Read the model definition and answer for the solid it produces. Units are mm, in the model's axes. Face numbers are marked on the shaded views. A direction names the side the tool comes from. Coordinates: 2 decimals unless noted, no trailing zeros. Loops run counter-clockwise (first coordinate to the right, second up) from the corner with the lowest first, then second, coordinate; pieces in that order, holes last.
from build123d import *

# Parameters (mm, degrees)
SKETCH_1_R          = 4.5
SKETCH_1_R_2        = 3
EXTRUDE_1_DEPTH     = 2
SKETCH_2_R          = 10
SKETCH_2_R_2        = 1.65
EXTRUDE_2_DEPTH     = 2.5
SKETCH_3_R          = 1.5
CUT_EXTRUDE_1_DEPTH = 2.5


with BuildPart() as part:
    # 草图1 → 凸台-拉伸1 (new body)
    with BuildSketch(Plane.XY):
        Circle(SKETCH_1_R)
        Circle(SKETCH_1_R_2, mode=Mode.SUBTRACT)
    extrude(amount=EXTRUDE_1_DEPTH)

    # 草图2 → 凸台-拉伸2 (add)
    with BuildSketch(Plane(origin=(0, 0, 0), x_dir=(-1, 0, 0), z_dir=(0, 0, -1))):
        Circle(SKETCH_2_R)
        Circle(SKETCH_2_R_2, mode=Mode.SUBTRACT)
    extrude(amount=EXTRUDE_2_DEPTH)

    # 草图3 → 切除-拉伸1 (cut)
    with BuildSketch(Plane(origin=(0, 0, -2.5), x_dir=(-1, 0, 0), z_dir=(0, 0, -1))):
        with Locations((7, 0)):
            Circle(SKETCH_3_R)
        with Locations((0, -7)):
            Circle(SKETCH_3_R)
        with Locations((-7, 0)):
            Circle(SKETCH_3_R)
        with Locations((0, 7)):
            Circle(SKETCH_3_R)
    extrude(amount=-CUT_EXTRUDE_1_DEPTH, mode=Mode.SUBTRACT)


solid = part.part
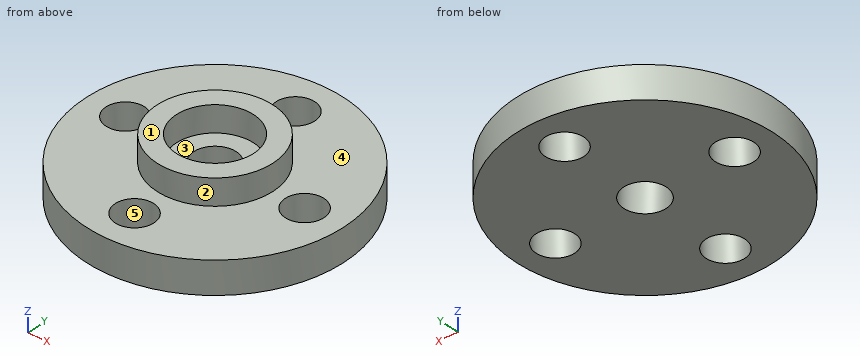
Item 1: A cutting plane is placed at B-B on y = 1.25. Determine the outline of the cut face in (x, z).
Numbers:
outline: (-9.92, -2.5) - (-7.83, -2.5) - (-7.83, 0) - (-9.92, 0) - close; (-6.17, -2.5) - (-1.08, -2.5) - (-1.08, 0) - (-2.73, 0) - (-2.73, 2) - (-4.32, 2) - (-4.32, 0) - (-6.17, 0) - close; (1.08, -2.5) - (6.17, -2.5) - (6.17, 0) - (4.32, 0) - (4.32, 2) - (2.73, 2) - (2.73, 0) - (1.08, 0) - close; (7.83, -2.5) - (9.92, -2.5) - (9.92, 0) - (7.83, 0) - close
Item 2: A cutting plane is placed at D-D on z = 0.4. Determine the outline of the cut face in (x, y).
Numbers:
outline: circle Ø9 at (0, 0); hole circle Ø6 at (0, 0)
Item 3: Given pin 1 (2 mm diameter, centred on x = 4, z = 0, fed in from +Y); pin 2 (4 mm diameter, centred on x = 6.5, y = 6.5, fed in from +Z); pin 3 (1.8 mm diameter, centred on x = -7, y = 0, fed in from -Z), each flat-ended and moving along its own axis, determine where each tip first touches the part or whether it passes through.
Numbers:
pin 1: stops at y = 9.54
pin 2: stops at z = 0
pin 3: passes through
Item 4: Determine the mould class of the marked faces 1, 2 and 3 for opening direction Y: released by +Y, released by -Y, zero draft, split by the parting line, or undercut.
Numbers:
face 1: zero draft
face 2: split by the parting line
face 3: undercut
Item 5: A cutting plane is placed at C-C on y = 7.5. Determine the outline of the cut face in (x, z).
Numbers:
outline: (-6.61, -2.5) - (-1.41, -2.5) - (-1.41, 0) - (-6.61, 0) - close; (1.41, -2.5) - (6.61, -2.5) - (6.61, 0) - (1.41, 0) - close
Item 6: A cutting plane is placed at A-A on x = 0. Determine the outline of the cut face in (y, z), then the cut area to 4 significant figures.
Numbers:
outline: (-10, -2.5) - (-8.5, -2.5) - (-8.5, 0) - (-10, 0) - close; (-5.5, -2.5) - (-1.65, -2.5) - (-1.65, 0) - (-3, 0) - (-3, 2) - (-4.5, 2) - (-4.5, 0) - (-5.5, 0) - close; (1.65, -2.5) - (5.5, -2.5) - (5.5, 0) - (4.5, 0) - (4.5, 2) - (3, 2) - (3, 0) - (1.65, 0) - close; (8.5, -2.5) - (10, -2.5) - (10, 0) - (8.5, 0) - close
area: 32.75 mm2
Item 7: Which of the six approach directions +Z, -Z, +X, -X, +Y, -Y give full straight-line access (tool end or side, diameter ignored) to the marked faces 4 and 5?
Numbers:
face 4: +Z
face 5: +Z, -Z
Item 8: Find the intervals of material crossed by line 1 along Y through (x, z) = (0, -1.35); line 2 along X through (y, z) = (-0.5, -1.3); line 3 along Z through (x, y) = (1.25, -8.75), in increasing order.
Numbers:
line 1: y = -10 to -8.5, -5.5 to -1.65, 1.65 to 5.5, 8.5 to 10
line 2: x = -9.99 to -8.41, -5.59 to -1.57, 1.57 to 5.59, 8.41 to 9.99
line 3: z = -2.5 to 0
